```python
from build123d import *

# Parameters (mm, degrees)
SKETCH1_W           = 130.2
SKETCH1_H           = 35
BOSS_EXTRUDE1_DEPTH = 2.4
SKETCH2_R           = 0.5
SKETCH2_R_2         = 3.625
CUT_EXTRUDE1_DEPTH  = 2.4
SKETCH6_W           = 0.5
SKETCH6_H           = 7.5
BOSS_EXTRUDE3_DEPTH = 0.5
FILLET3_R           = 15


with BuildPart() as part:
    # Sketch1 → Boss-Extrude1 (new body)
    with BuildSketch(Plane(origin=(0, 0, 0), x_dir=(1, 0, 0), z_dir=(0, 1, 0))):
        with Locations((62.422946176, 21.495750708)):
            Rectangle(SKETCH1_W, SKETCH1_H)
    extrude(amount=BOSS_EXTRUDE1_DEPTH)

    # Sketch2 → Cut-Extrude1 (cut)
    with BuildSketch(Plane(origin=(0, 2.4, 0), x_dir=(1, 0, 0), z_dir=(0, 1, 0))):
        with Locations(Location((16.807946176, 27.930319458, 0), (0, 0, 270))):
            Circle(SKETCH2_R)
        with Locations(Location((15.340446176, 30.472104018, 0), (0, 0, 270))):
            Circle(SKETCH2_R)
        with Locations(Location((13.837946176, 33.074510357, 0), (0, 0, 270))):
            Circle(SKETCH2_R)
        with Locations(Location((24.237946176, 27.930319458, 0), (0, 0, 270))):
            Circle(SKETCH2_R)
        with Locations(Location((20.522946176, 21.495750708, 0), (0, 0, 270))):
            Circle(SKETCH2_R_2)
        with Locations(Location((13.092946176, 21.495750708, 0), (0, 0, 270))):
            Circle(SKETCH2_R)
        with Locations(Location((10.157946176, 21.495750708, 0), (0, 0, 270))):
            Circle(SKETCH2_R)
        with Locations(Location((7.152946176, 21.495750708, 0), (0, 0, 270))):
            Circle(SKETCH2_R)
        with Locations(Location((25.705446176, 30.472104018, 0), (0, 0, 270))):
            Circle(SKETCH2_R)
        with Locations(Location((27.207946176, 33.074510357, 0), (0, 0, 270))):
            Circle(SKETCH2_R)
        with Locations(Location((27.952946176, 21.495750708, 0), (0, 0, 270))):
            Circle(SKETCH2_R)
        with Locations(Location((30.887946176, 21.495750708, 0), (0, 0, 270))):
            Circle(SKETCH2_R)
        with Locations(Location((33.892946176, 21.495750708, 0), (0, 0, 270))):
            Circle(SKETCH2_R)
        with Locations(Location((24.237946176, 15.061181958, 0), (0, 0, 270))):
            Circle(SKETCH2_R)
        with Locations(Location((25.705446176, 12.519397398, 0), (0, 0, 270))):
            Circle(SKETCH2_R)
        with Locations(Location((27.207946176, 9.91699106, 0), (0, 0, 270))):
            Circle(SKETCH2_R)
        with Locations(Location((16.807946176, 15.061181958, 0), (0, 0, 270))):
            Circle(SKETCH2_R)
        with Locations(Location((15.340446176, 12.519397398, 0), (0, 0, 270))):
            Circle(SKETCH2_R)
        with Locations(Location((13.837946176, 9.91699106, 0), (0, 0, 270))):
            Circle(SKETCH2_R)
    extrude(amount=-CUT_EXTRUDE1_DEPTH, mode=Mode.SUBTRACT)

    # Sketch6 → Boss-Extrude3 (add)
    with BuildSketch(Plane(origin=(0, 2.4, 0), x_dir=(1, 0, 0), z_dir=(0, 1, 0))):
        with Locations((20.522946176, 7.745750708)):
            Rectangle(SKETCH6_W, SKETCH6_H)
        with Locations((20.522946176, 35.245750708)):
            Rectangle(SKETCH6_W, SKETCH6_H)
    extrude(amount=BOSS_EXTRUDE3_DEPTH)

    # Fillet3
    fillet3_edges = [part.edges().sort_by_distance(p)[0] for p in [
        (-2.677053824, 1.2, -38.995750708),
        (-2.677053824, 1.2, -3.995750708),
    ]]
    fillet(fillet3_edges, radius=FILLET3_R)


solid = part.part
```
The listing builds one solid part. Answer for the finished solid, in the listing's coordinates (mm). Coordinates: 2 decimals unless noted, no trailing zeros. Write each loop counter-clockwise with the first axis right and the second up, starting at its lowest first coordinate (ties: lowest second). Pieces come first, ordered by that corner, then holes. Notation, with made-up numbers: (59.5, 15) - (67.5, 15) arc R27 ccw to (67.5, 51) - close; hole circle Ø5 at (19, 72.5). An arc over 180 degrees is marked (long way). Return JSON: item names as keys, results as strings. Group by question number.
1. A cutting plane is placed at C-C, the plane x = 76. Determine the outline of the cut face in (y, z).
2. Straight lines are drawn through the part: L1, parallel to X at y = 2.2, z = -27.5; L2, parallel to Y at x = 16, z = -34; L3, parallel to X at y = 2.45, z = -10. For each, find the intervals that lie inside material, in ascending order.
3. Determine the mould class of faces 1 (the flat face through (69, 1, -3.996)), 2 (the cylindrical face through (1.6, 1.217, -34.485)), 3 (the cylindrical face through (18.317, 1.217, -24.372)) for opening direction X: released by +X, released by -X, zero draft, split by the parting line, or undercut.
4. A cutting plane is placed at B-B, the plane z = -35.5. Determine the outline of the cut face in (x, y), plus the area to 3 significant figures.
5. Given pin 1 (8 mm diameter, centred on x = 88.5, z = -31, fed in from +Y); pin 2 (2 mm diameter, centred on x = 41, z = -23.5, fed in from -Y), each flat-ended and moving along its own axis, determine where each tip first touches the part or whether it passes through.
6. A cutting plane is placed at A-A, the plane y = 0.5. Give the number of separate pieces and of enclosed holes in the cut face, plus the area to 4 significant figures.
Ans:
{
 "1": {"outline": "(0, -39) - (2.4, -39) - (2.4, -4) - (0, -4) - close"},
 "2": {"L1": "-2.26 to 16.55, 17.06 to 23.98, 24.49 to 127.52", "L2": "0 to 2.4", "L3": "20.27 to 20.77"},
 "3": {"face 1": "zero draft", "face 2": "released by -X", "face 3": "undercut"},
 "4": {"outline": "(2.7, 0) - (127.52, 0) - (127.52, 2.4) - (20.77, 2.4) - (20.77, 2.9) - (20.27, 2.9) - (20.27, 2.4) - (2.7, 2.4) - close", "area": "300 mm²"},
 "5": {"pin 1": "y = 2.4", "pin 2": "y = 0"},
 "6": {"separate pieces": "1", "enclosed holes": "19", "area": "4,405 mm²"}
}
